Could you check a few things on this model? Use its own coordinates, in mm. A direction names the side the tool comes from. Round coordinates to 2 decimals unless told otherwise and drop trailing zeros. Loops run counter-clockwise (first coordinate to the right, second up) from the corner with the lowest first, then second, coordinate; pieces in that order, holes last. Notation, with made-up numbers: (55.25, 3.25) -> (104.25, 3.25) arc R12 ccw to (104.25, 26.25) -> close; hole circle Ø11 at (-35, -33). An arc over 180 degrees is marked (long way). Use CSV: the item, a comma, the result in double quotes. Start each with the question number.
Autodesk Inventor part; units mm, degrees
ref_plane "YZ Plane" through (0, 0, 0) normal (1, 0, 0) x (0, 1, 0)
ref_plane "XZ Plane" through (0, 0, 0) normal (0, 1, 0) x (-1, 0, 0)
ref_plane "XY Plane" through (0, 0, 0) normal (0, 0, 1) x (1, 0, 0)
sketch "Sketch1" plane through (0, 0, 0) normal (0, 1, 0) x (-1, 0, 0)
  circle A0 centre (0, 0) radius 31.75
  dimension "od" = 63.5
extrude "Extrusion1" add sketch "Sketch1" against normal blind 3.556
sketch "Sketch3" plane through (0, -3.556, 0) normal (0, -1, 0) x (1, 0, 0)
  circle A0 centre (0, 0) radius 13.589
  dimension "idWasher" = 27.178
extrude "Extrusion3" add sketch "Sketch3" along normal blind 2.54
sketch "Sketch2" plane through (0, 0, 0) normal (0, 1, 0) x (1, 0, 0)
  line L0 (-7.7063, 0) -> (-3.8531, 6.6738)
  line L1 (-3.8531, 6.6738) -> (3.8531, 6.6738)
  line L2 (3.8531, 6.6738) -> (7.7063, 0)
  line L3 (7.7063, 0) -> (3.8531, -6.6738)
  line L4 (3.8531, -6.6738) -> (-3.8531, -6.6738)
  line L5 (-3.8531, -6.6738) -> (-7.7063, 0)
  point P0 (0, 0)
  point P1 (0, 0)
  dimension "d3" = 13.3477
extrude "Extrusion2" cut sketch "Sketch2" against normal through all
chamfer "Chamfer1" distance 1.5875 angle 45 12 edges at (-5.7797, 0, -3.3369) (0, 0, -6.6738) (5.7797, 0, -3.3369) (5.7797, 0, 3.3369) (0, 0, 6.6738) (-5.7797, 0, 3.3369) (5.7797, -6.096, -3.3369) (5.7797, -6.096, 3.3369) (0, -6.096, 6.6738) (-5.7797, -6.096, 3.3369) (-5.7797, -6.096, -3.3369) (0, -6.096, -6.6738)
properties part number "spacerForEnd" material "PC/ABS Plastic"
1. Suppose I cut it at C-C (x = -6.5). List the corners of the cut face in (y, z) for me.
2. Suppose I cut it at A-A (x = 0). List the corners of the cut face in (y, z) for me, then the cut area to 3 significant figures.
3. Suppose I cut it at B-B (y = -2.5). List the corners of the cut face in (x, z) for me, then the cut area to 3 significant figures.
4. For faces 4 (the face through (-7, 0, -7)), 5 (the face through (-5.753, -3.028, 3.384)), 6 (the face through (0.07, -0.8, -7.46)), 7 (the face through (-6.51, -5.31, 3.68)), which set-ups out of +Z, -Z, +X, -X, +Y, -Y let a thin tool reach every point of the face, with its end or its side?
5. We'd pull the mould along X, two halves only. Please class faces 1 (the face through (0, -3, -6.674)), 2 (the face through (12.96, -4.81, -4.08)), 3 (the face through (0, -6.096, -9)): pulls with the +X half, pulls with the -X half, needs draft (parallel to the pull), parting line crosses it, or undercut.
6. Will these pins go through, and if not, where does the flat tip stop? pin 1 (3 mm diameter, centred on x = 1.5, y = -3.5, fed in from +Z); pin 2 (3 mm diameter, centred on y = -1.5, z = -2, fed in from -X); pin 3 (1 mm diameter, centred on x = 12, z = -18.5, fed in from -Y).
7. If I drill on L1, parallel to Y at x = -27, z = -11; L2, parallel to Z at x = -3, y = -3; L3, parallel to X at y = -3.5, z = 28, over which ranges is the centre line in solid material (lowest first)?
8. Suppose I cut it at D-D (z = -18). List the corners of the cut face in (x, y) for me, then the cut area to 3 significant figures.
Geometry check:
1,outline,"(-6.1, -11.93) -> (-3.56, -11.93) -> (-3.56, -31.08) -> (0, -31.08) -> (0, -5.26) -> (-1.59, -2.09) -> (-4.51, -2.09) -> (-6.1, -5.26) -> close; (-6.1, 5.26) -> (-4.51, 2.09) -> (-1.59, 2.09) -> (0, 5.26) -> (0, 31.08) -> (-3.56, 31.08) -> (-3.56, 11.93) -> (-6.1, 11.93) -> close"
2,outline,"(-6.1, -13.59) -> (-3.56, -13.59) -> (-3.56, -31.75) -> (0, -31.75) -> (0, -8.26) -> (-1.59, -6.67) -> (-4.51, -6.67) -> (-6.1, -8.26) -> close; (-6.1, 8.26) -> (-4.51, 6.67) -> (-1.59, 6.67) -> (0, 8.26) -> (0, 31.75) -> (-3.56, 31.75) -> (-3.56, 13.59) -> (-6.1, 13.59) -> close"
2,area,"208 mm²"
3,outline,"circle Ø63.5 at (0, 0); hole (-7.71, 0) -> (-3.85, -6.67) -> (3.85, -6.67) -> (7.71, 0) -> (3.85, 6.67) -> (-3.85, 6.67) -> close"
3,area,"3,010 mm²"
4,face 4,"+Z, -Z, +X, -X, +Y"
4,face 5,"+Y, -Y"
4,face 6,"+Y"
4,face 7,"-Y"
5,face 1,"undercut"
5,face 2,"parting line crosses it"
5,face 3,"needs draft"
6,pin 1,"stops at z = 31.75"
6,pin 2,"stops at x = -31.75"
6,pin 3,"stops at y = -3.56"
7,L1,"y = -3.56 to 0"
7,L2,"z = -31.61 to -6.67, 6.67 to 31.61"
7,L3,"x = -14.97 to 14.97"
8,outline,"(-26.15, -3.56) -> (26.15, -3.56) -> (26.15, 0) -> (-26.15, 0) -> close"
8,area,"186 mm²"
